from build123d import *

# Parameters (mm, degrees)
EXTRUDE_1_DEPTH     = 45
FILLET_1_R          = 2
SKETCH_2_R          = 15
CUT_EXTRUDE_1_DEPTH = 10
FILLET_2_R          = 2
SKETCH_4_R          = 1.65
CUT_EXTRUDE_2_DEPTH = 10
SKETCH_5_R          = 1.5
CUT_EXTRUDE_3_DEPTH = 10


with BuildPart() as part:
    # 草图1 → 拉伸-薄壁1 (new body)
    with BuildSketch(Plane(origin=(0, 0, 0), x_dir=(1, 0, 0), z_dir=(0, 1, 0))):
        Polygon((0, 0), (0, 48.91), (45, 48.91), (45, 46.91), (2, 46.91), (2, 0), align=None)
    extrude(amount=EXTRUDE_1_DEPTH)

    # 圆角1
    fillet_1_edges = [part.edges().sort_by_distance(p)[0] for p in [
        (2, 22.5, -46.91),
        (0, 22.5, -48.91),
    ]]
    fillet(fillet_1_edges, radius=FILLET_1_R)

    # 草图2 → 切除-拉伸1 (cut)
    with BuildSketch(Plane.ZY):
        with Locations((-22.5, 22.5)):
            Circle(SKETCH_2_R)
    extrude(amount=-CUT_EXTRUDE_1_DEPTH, mode=Mode.SUBTRACT)

    # 圆角2
    fillet_2_edges = [part.edges().sort_by_distance(p)[0] for p in [
        (1, 45, 0),
        (1, 0, 0),
        (45, 0, -47.91),
        (45, 45, -47.91),
    ]]
    fillet(fillet_2_edges, radius=FILLET_2_R)

    # 草图4 → 切除-拉伸2 (cut)
    with BuildSketch(Plane.ZY):
        with Locations((-34.874368671, 10.125631329)):
            Circle(SKETCH_4_R)
        with Locations((-10.125631329, 10.125631329)):
            Circle(SKETCH_4_R)
        with Locations((-10.125631329, 34.874368671)):
            Circle(SKETCH_4_R)
        with Locations((-34.874368671, 34.874368671)):
            Circle(SKETCH_4_R)
    extrude(amount=-CUT_EXTRUDE_2_DEPTH, mode=Mode.SUBTRACT)

    # 草图5 → 切除-拉伸3 (cut)
    with BuildSketch(Plane.XY.offset(-46.91)):
        with Locations((12.5, 35)):
            Circle(SKETCH_5_R)
        with Locations((37.5, 35)):
            Circle(SKETCH_5_R)
    extrude(amount=-CUT_EXTRUDE_3_DEPTH, mode=Mode.SUBTRACT)


solid = part.part
Can you work these out from the model? Positions are in its coordinate system, mm. A direction names the side the tool comes from. Coordinates: 2 decimals unless noted, no trailing zeros. Write each loop counter-clockwise with the first axis right and the second up, starting at its lowest first coordinate (ties: lowest second). Pieces come first, ordered by that corner, then holes. Notation, with made-up numbers: (6, 21) -> (47, 21) arc R19 ccw to (47, 33) -> close; hole circle Ø7 at (-23, 89). An arc over 180 degrees is marked (long way). Write each question's results on one line, items separated by ' | '. Start each with the question number.
Q1. Imagine slicing it at C-C (x = 37.5). Write out the boundary of the cut face in (y, z).
Q2. We'd pull the mould along X, two halves only. Please class faces 3 (the face through (2.6, 22.82, -46.34)), 4 (the face through (0.986, 10.198, -11.774)), 5 (the face through (0, 12, -34)), 6 (the face through (36.3, 34.1, -47.9)): +X half, -X half, draft (parallel to the pull), parting line (faces both ways), or undercut.
Q3. Imagine slicing it at D-D (z = -41.5). Write out the boundary of the cut face in (x, y).
Q4. If I drill on probe 1 along Y at (x, z) = (12.5, -47.45); probe 2 along Y at (x, z) = (1.2, -22.5); probe 3 along Z at (x, y) = (36, 8), over which ranges is the centre line in solid material (lowest first)?
Q5. Imagine slicing it at A-A (z = -22.5). Write out the boundary of the cut face in (x, y).
Q6. Imagine slicing it at B-B (y = 22.5). Write out the boundary of the cut face in (x, z).
Q7. I'm going to push flat-ended pins straight in: pin 1 (5 mm diameter, centred on x = 12.5, y = 35, fed in from +Z); pin 2 (4.5 mm diameter, centred on y = 10.13, z = -34.87, fed in from +X). Where does each tip first touch, or does it pass through?
Q8. On a 3-axis mill with a long thin cutter (end or side, diameter ignored), from which of +Z, -Z, +X, -X, +Y, -Y can I reach the whole of each face in a straight line? I mean faces 1 (the face through (25, 22, -46.91)), 2 (the face through (12.175, 33.536, -47.896)). Say none if no direction works.
Taken from the geometry:
1) outline: (0, -48.91) -> (33.5, -48.91) -> (33.5, -46.91) -> (0, -46.91) -> close; (36.5, -48.91) -> (45, -48.91) -> (45, -46.91) -> (36.5, -46.91) -> close
2) face 3: +X half | face 4: draft | face 5: -X half | face 6: undercut
3) outline: (0, 0) -> (2, 0) -> (2, 45) -> (0, 45) -> close
4) probe 1: y = 0 to 33.5, 36.5 to 45 | probe 2: y = 0 to 7.5, 37.5 to 45 | probe 3: z = -48.91 to -46.91
5) outline: (0, 0) -> (2, 0) -> (2, 7.5) -> (0, 7.5) -> close; (0, 37.5) -> (2, 37.5) -> (2, 45) -> (0, 45) -> close
6) outline: (0, -46.91) arc R2 ccw to (2, -48.91) -> (45, -48.91) -> (45, -46.91) -> (4, -46.91) arc R2 cw to (2, -44.91) -> (2, -37.5) -> (0, -37.5) -> close; (0, -7.5) -> (2, -7.5) -> (2, 0) -> (0, 0) -> close
7) pin 1: stops at z = -46.91 | pin 2: stops at x = 2
8) face 1: +Z, +X, +Y, -Y | face 2: +Z, -Z
